Geometry check sheet. Reference: the model listing, model coordinates, mm. A direction names the side the tool comes from. Round coordinates to 2 decimals unless told otherwise and drop trailing zeros. Write each loop counter-clockwise with the first axis right and the second up, starting at its lowest first coordinate (ties: lowest second). Pieces come first, ordered by that corner, then holes. Notation, with made-up numbers: M -37.5,38 L 21.5,38 A21 ccw 21.5,59 Z; hole C -10.75,82 d11. An arc over 180 degrees is marked long. Use a Markdown table: item, result.
Autodesk Inventor part; units mm, degrees
ref_plane "Work Plane1" through (29, 0, 0) normal (0, -1, 0) x (1, 0, 0)
ref_plane "YZ Plane" through (0, 0, 0) normal (1, 0, 0) x (0, 1, 0)
ref_plane "XZ Plane" through (0, 0, 0) normal (0, 1, 0) x (-1, 0, 0)
sketch "Sketch1" plane through (0, 0, 0) normal (0, 0, 1) x (1, 0, 0)
  line L0 (-0.7535, 0) -> (6.35, 0)
  line L1 (6.35, 0) -> (6.35, 1.4224)
  line L2 (6.35, 1.4224) -> (1.5877, 1.4224)
  line L3 (1.5877, 1.4224) -> (0.0001, 1.4224)
  line L4 (0.0001, 1.4224) -> (0, 1.4224)
  line L5 (0, 1.4224) -> (0, 2.3241)
  line L6 (0, 2.3241) -> (-2.8448, 2.3241)
  line L7 (-2.8448, 2.3241) -> (-2.8448, 1.3785)
  line L8 (-2.8448, 1.3785) -> (-1.5494, 1.3785)
  line L9 (-1.5494, 1.3785) -> (-0.7535, 0)
  line L10 (-4.6838, 0) -> (8.189, 0)
  line L11 (0, -0.4648) -> (0, 2.7889)
  line L12 (1.5877, 1.4224) -> (0, 1.4224) construction
  dimension "d1" = 4.7623
  dimension "d2" = 1.5876
  dimension "d3" = 2.8448
  dimension "d4" = 1.2954
  dimension "d5" = 60
  dimension "d6" = 2.8448
  dimension "d7" = 2.8448
  dimension "d8" = 2.757
  dimension "d9" = 4.6482
  dimension "d26" = 6.35
revolve "Body" add sketch "Sketch1" angle 360 about axis through (-0.7535, 0, 0) along (1, 0, 0)
sketch "Sketch2" plane through (-2.8448, 0, 0) normal (-1, 0, 0) x (0, 0, 1)
  circle A0 centre (0, 0) radius 1.3785
  line L0 (0, -3.2537) -> (0, 3.2537)
  line L1 (-3.2537, 0) -> (3.2537, 0)
  line L2 (1.3785, 0) -> (0.6892, -1.1938)
  line L3 (0.6892, -1.1938) -> (-0.6892, -1.1938)
  line L4 (-0.6892, -1.1938) -> (-1.3785, 0)
  line L5 (-1.3785, 0) -> (-0.6892, 1.1938)
  line L6 (-0.6892, 1.1938) -> (0.6892, 1.1938)
  line L7 (0.6892, 1.1938) -> (1.3785, 0)
  point P0 (0, 0)
extrude "Slot" add sketch "Sketch2" against normal up to next contours L7 A0 | A0 L2 | L6 L0 A0 | A0 L0 L3 | L0 L6 A0 | A0 L3 L0 | L4 A0 | A0 L5
fillet "Fillet1" radius 0.2286 1 edges at (-2.8448, -2.3241, 0)
thread "Thread"
chamfer "Chamfer1" distance 0.3785 distance2 0.3785 1 edges at (6.35, -1.4224, 0) measured on face at (6.35, -0.0627, 0.6443)
ref_plane "Work Plane1" through (29, 0, 0) normal (0, -1, 0) x (1, 0, 0)
fillet "Fillet2" radius 0.1016 1 edges at (0.0001, -1.4224, 0)
equation "\"d1\" = GEL"
equation "\"d3\" = KOH"
equation "\"d4\" = INTI"
equation "\"d6\" = GD"
equation "\"d7\" = BDM"
equation "\"d8\" = 1.1547 * SW"
equation "\"d9\" = KOD"
equation "\"d26\" = NLG"
equation "\"d30\" = R"
equation "\"d17\" = RR"
equation "\"d13\" = GEL"
equation "\"d15\" = -0.5 * SPD + 0.5 * GD"
equation "\"d16\" = GUL"
equation "\"GD\" = 2.8448"
equation "\"NLG\" = 6.35"
equation "\"GEL\" = 4.7623"
equation "\"KOD\" = 4.6482"
equation "\"KOH\" = 2.8448"
equation "\"INTI\" = 1.2954"
equation "\"GAL\" = 1.5875"
equation "\"GUL\" = 0.37846"
equation "\"BDM\" = 2.8448"
equation "\"SW\" = 2.3876"
equation "\"RR\" = 0.2286"
equation "\"SPD\" = 2.08788"
equation "\"R\" = 0.1016"
equation "\"PHH\" = 0.127"
equation "\"GD1\" = SPD"
equation "\"THREADDIA\" = 2.8448"
equation "\"FAWI\" = 45deg"
equation "\"KOH1\" = 2.5654"
equation "\"NND\" = 2.8448"
equation "\"TOA\" = 30deg"
equation "\"E0\" = 1.155 * SW"
properties part number "ANSI B18.3 - No. 4 - 40 UNC - 1/4 HS HCS" material "Steel, Mild"
Item 1: Material ranges on line 1 along Z through (x, y) = (4, 0.05); line 2 along Z through (x, y) = (-2, -0.3), recorded low to high. Write a range as from..to.
Outcome:
| item | result |
|---|---|
| line 1 | z = -1.42..1.42 |
| line 2 | z = -2.3..-1.21, 1.21..2.3 |
Item 2: Cross-section at A-A, the plane x = 5.5. Record the cut outline in (y, z).
Outcome:
| item | result |
|---|---|
| outline | C 0,0 d2.84 |
Item 3: Access from +Z, -Z, +X, -X, +Y, -Y to the whole of each face (thin tool, end or side, straight path). Record for faces 4 (the face through (-2.154, -0.605, -1.029)), 5 (the face through (0, 2, 0)), 6 (the face through (-1.33, -0.5, 2.27)).
Outcome:
| item | result |
|---|---|
| face 4 | -X |
| face 5 | +X |
| face 6 | +X, -X |
Item 4: Mould release check, pull along Z, two halves, no side actions. Record for faces 1 (the face through (3, -1.1, 0.9)), 2 (the face through (-2.845, -1, 1)), 3 (the face through (-0.803, -0.011, -0.085)): +Z half, -Z half, draft (parallel to the pull), parting line (faces both ways), or undercut.
Outcome:
| item | result |
|---|---|
| face 1 | parting line |
| face 2 | draft |
| face 3 | undercut |
